Source: CAD feature listing. Evaluate the final solid. Frame: model axes, mm. A direction names the side the tool comes from. Round coordinates to 2 decimals unless told otherwise and drop trailing zeros. Loops run counter-clockwise (first coordinate to the right, second up) from the corner with the lowest first, then second, coordinate; pieces in that order, holes last.
Item 1: Section query A-A on x = 0. Return loops of the section in (y, z).
Item 2: Ray query, L1, parallel to Y at x = 0, z = 0.25; L2, parallel to Z at x = 13, y = -36; L3, parallel to X at y = 35, z = 2.5. Return the intervals inside material, ascending.
Item 3: Pull-direction query (X, two-part tool) for faces 1 (the cylindrical face through (-18.114, -31.111, -3.507)), 2 (the flat face through (-14, -4, 5)), 3 (the cylindrical face through (12.932, -5.362, -0.07)); classes: released by +X, released by -X, zero draft, split by the parting line, or undercut.
Item 4: Access query for faces 4 (the cylindrical face through (18.114, 31.111, 3.493)), 5 (the flat face through (20, -20, 0)), 6 (the cylindrical face through (18.114, 31.111, -3.507)), 7 (the flat face through (25, -41, -3)), 8 (the flat face through (-13, -24, 4)). Directions: +Z, -Z, +X, -X, +Y, -Y. A direction counts if a zero-diameter tool reaches every point of the face in a straight line with its end or side. Return the directions, or none.
Item 5: Section query C-C on y = -22. Return loops of the section in (x, z).
Item 6: First-contact query: P1, Ø2, axis at x = 21, z = 3, coming from the +Y side; P2, Ø5, axis at x = 26.5, y = -2.5, coming from the -Z side; P3, Ø3, axis at x = -47, y = 8.5, coming from the -Z side; P4, Ø9.5, axis at x = -44.5, y = 4.5, coming from the +Z side. Flat tips, straight axial feed; report the tip coordinate or a pass-through.
Item 7: Section query D-D on x = 33. Return loops of the section in (y, z).
```python
from build123d import *

# Parameters (mm, degrees)
SKETCH1_R           = 20
SKETCH1_R_2         = 14
BOSS_EXTRUDE1_DEPTH = 5
BOSS_EXTRUDE2_DEPTH = 4
BOSS_EXTRUDE3_DEPTH = 3


with BuildPart() as part:
    # Sketch1 → Boss-Extrude1 (new, symmetric)
    with BuildSketch(Plane.XY):
        Circle(SKETCH1_R)
        Circle(SKETCH1_R_2, mode=Mode.SUBTRACT)
    extrude(amount=BOSS_EXTRUDE1_DEPTH, both=True)

    # Sketch1_3 → Boss-Extrude2 (add, symmetric)
    with BuildSketch(Plane.XY):
        with BuildLine():
            ThreePointArc((-14.142135624, 14.142135624), (-10, 17.320508076), (-5.176380902, 19.318516526))
            Line((-5.176380902, 19.318516526), (-9.317485624, 34.773329746))
            ThreePointArc((-9.317485624, 34.773329746), (-18, 31.176914536), (-25.455844123, 25.455844123))
            Line((-25.455844123, 25.455844123), (-14.142135624, 14.142135624))
        make_face()
        with BuildLine():
            ThreePointArc((5.176380902, 19.318516526), (10, 17.320508076), (14.142135624, 14.142135624))
            Line((14.142135624, 14.142135624), (25.455844123, 25.455844123))
            ThreePointArc((25.455844123, 25.455844123), (18, 31.176914536), (9.317485624, 34.773329746))
            Line((9.317485624, 34.773329746), (5.176380902, 19.318516526))
        make_face()
        with BuildLine():
            Line((34.773329746, 9.317485624), (19.318516526, 5.176380902))
            ThreePointArc((19.318516526, 5.176380902), (19.828897227, 2.610523844), (20, 0))
            ThreePointArc((20, 0), (19.828897227, -2.610523844), (19.318516526, -5.176380902))
            Line((19.318516526, -5.176380902), (34.773329746, -9.317485624))
            ThreePointArc((34.773329746, -9.317485624), (36, 0), (34.773329746, 9.317485624))
        make_face()
        with BuildLine():
            Line((25.455844123, -25.455844123), (14.142135624, -14.142135624))
            ThreePointArc((14.142135624, -14.142135624), (10, -17.320508076), (5.176380902, -19.318516526))
            Line((5.176380902, -19.318516526), (9.317485624, -34.773329746))
            ThreePointArc((9.317485624, -34.773329746), (18, -31.176914536), (25.455844123, -25.455844123))
        make_face()
        with BuildLine():
            Line((-9.317485624, -34.773329746), (-5.176380902, -19.318516526))
            ThreePointArc((-5.176380902, -19.318516526), (-10, -17.320508076), (-14.142135624, -14.142135624))
            Line((-14.142135624, -14.142135624), (-25.455844123, -25.455844123))
            ThreePointArc((-25.455844123, -25.455844123), (-18, -31.176914536), (-9.317485624, -34.773329746))
        make_face()
        with BuildLine():
            ThreePointArc((-19.318516526, -5.176380902), (-20, 0), (-19.318516526, 5.176380902))
            Line((-19.318516526, 5.176380902), (-34.773329746, 9.317485624))
            ThreePointArc((-34.773329746, 9.317485624), (-36, 0), (-34.773329746, -9.317485624))
            Line((-34.773329746, -9.317485624), (-19.318516526, -5.176380902))
        make_face()
    extrude(amount=BOSS_EXTRUDE2_DEPTH, both=True)

    # Sketch1_4 → Boss-Extrude3 (add, symmetric)
    with BuildSketch(Plane.XY):
        with BuildLine():
            ThreePointArc((-9.317485624, 34.773329746), (-18, 31.176914536), (-25.455844123, 25.455844123))
            Line((-25.455844123, 25.455844123), (-36.5, 63.219854476))
            Line((-36.5, 63.219854476), (-9.317485624, 34.773329746))
        make_face()
        with BuildLine():
            ThreePointArc((25.455844123, 25.455844123), (18, 31.176914536), (9.317485624, 34.773329746))
            Line((9.317485624, 34.773329746), (36.5, 63.219854476))
            Line((36.5, 63.219854476), (25.455844123, 25.455844123))
        make_face()
        with BuildLine():
            ThreePointArc((34.773329746, -9.317485624), (36, 0), (34.773329746, 9.317485624))
            Line((34.773329746, 9.317485624), (73, 0))
            Line((73, 0), (34.773329746, -9.317485624))
        make_face()
        with BuildLine():
            ThreePointArc((9.317485624, -34.773329746), (18, -31.176914536), (25.455844123, -25.455844123))
            Line((25.455844123, -25.455844123), (36.5, -63.219854476))
            Line((36.5, -63.219854476), (9.317485624, -34.773329746))
        make_face()
        with BuildLine():
            ThreePointArc((-25.455844123, -25.455844123), (-18, -31.176914536), (-9.317485624, -34.773329746))
            Line((-9.317485624, -34.773329746), (-36.5, -63.219854476))
            Line((-36.5, -63.219854476), (-25.455844123, -25.455844123))
        make_face()
        with BuildLine():
            ThreePointArc((-34.773329746, 9.317485624), (-36, 0), (-34.773329746, -9.317485624))
            Line((-34.773329746, -9.317485624), (-73, 0))
            Line((-73, 0), (-34.773329746, 9.317485624))
        make_face()
    extrude(amount=BOSS_EXTRUDE3_DEPTH, both=True)


solid = part.part
```
Data:
1. outline: (-20, -5) - (-14, -5) - (-14, 5) - (-20, 5) - close; (14, -5) - (20, -5) - (20, 5) - (14, 5) - close
2. L1: y = -20 to -14, 14 to 20
2. L2: z = -3 to 3
2. L3: x = -28.25 to -9.53, 9.53 to 28.25
3. face 1: released by -X
3. face 2: zero draft
3. face 3: undercut
4. face 4: +Z, +X, +Y
4. face 5: +Z, -Z, +X
4. face 6: -Z, +X, +Y
4. face 7: -Z, +X, -Y
4. face 8: +Z, -X, -Y
5. outline: (-22, -4) - (-5.89, -4) - (-5.89, 4) - (-22, 4) - close; (5.89, -4) - (22, -4) - (22, 4) - (5.89, 4) - close
6. P1: stops at y = 48.05
6. P2: stops at z = -4
6. P3: passes through
6. P4: stops at z = 3
7. outline: (-59.56, -3) - (-51.25, -3) - (-51.25, 3) - (-59.56, 3) - close; (-8.84, -4) - (8.84, -4) - (8.84, 4) - (-8.84, 4) - close; (51.25, -3) - (59.56, -3) - (59.56, 3) - (51.25, 3) - close
